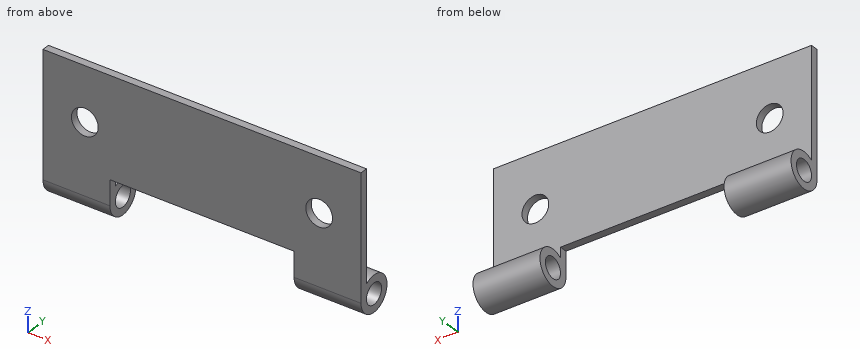
from build123d import *

# Parameters (mm, degrees)
SKETCH_1_R          = 1.25
EXTRUDE_1_DEPTH     = 38
SKETCH_2_R          = 1.6
SKETCH_2_W          = 22
SKETCH_2_H          = 7.890130192
CUT_EXTRUDE_1_DEPTH = 19


with BuildPart() as part:
    # 草图1 → 凸台-拉伸1 (new body)
    with BuildSketch(Plane(origin=(0, 0, 0), x_dir=(0, 0, -1), z_dir=(1, 0, 0))):
        with BuildLine():
            Line((0, -2.15), (-15, -2.15))
            Line((-15, -2.15), (-15, -1.25))
            Line((-15, -1.25), (-1.749285568, -1.25))
            ThreePointArc((-1.749285568, -1.25), (0.983615779, 1.911805429), (0, -2.15))
        make_face()
        Circle(SKETCH_1_R, mode=Mode.SUBTRACT)
    extrude(amount=EXTRUDE_1_DEPTH)

    # 草图2 → 切除-拉伸1 (cut, symmetric)
    with BuildSketch(Plane(origin=(0, 0, 0), x_dir=(1, 0, 0), z_dir=(0, 1, 0))):
        with Locations((33, -8.5)):
            Circle(SKETCH_2_R)
        with Locations((5, -8.5)):
            Circle(SKETCH_2_R)
        with Locations((19, 0.945065096)):
            Rectangle(SKETCH_2_W, SKETCH_2_H)
    extrude(amount=CUT_EXTRUDE_1_DEPTH, both=True, mode=Mode.SUBTRACT)


solid = part.part
Verification items for the finished model (mm, model axes). Give positions to 0.01 mm unless a question says otherwise; leave off trailing zeros. Write each loop counter-clockwise with the first axis right and the second up, starting at its lowest first coordinate (ties: lowest second). Pieces come first, ordered by that corner, then holes. Notation, with made-up numbers: (28.5, 72.25) - (73.5, 72.25) arc R21 ccw to (73.5, 103.25) - close; hole circle Ø8 at (-11.75, 63.5). An arc over 180 degrees is marked (long way). Answer as CSV lines item,"result". Start each with the question number.
1. Sectioned sample at C-C (z = 8.5). Record the boundary of the cut face in (x, y), then the cut area to 3 significant figures.
2. Depth check by flat-ended pin: pin 1 (6 mm diameter, centred on x = 12, z = 6.5, fed in from +Y). Enter the tip coordinate at first touch or a pass-through.
3. Sectioned sample at B-B (y = 0). Record the boundary of the cut face in (x, z).
4. Thickness scan on line 1 (Z direction, x = 36.25, y = 0); line 2 (Z direction, x = 5, y = -1.75); line 3 (Z direction, x = 20, y = -1.6). Record the ranges inside material, lowest first.
5. Sectioned sample at D-D (y = -1.7). Record the boundary of the cut face in (x, z).
6. Sectioned sample at A-A (x = 33). Record the boundary of the cut face in (y, z), then the cut area to 3 significant figures.
Derived:
1,outline,"(0, -2.15) - (3.4, -2.15) - (3.4, -1.25) - (0, -1.25) - close; (6.6, -2.15) - (31.4, -2.15) - (31.4, -1.25) - (6.6, -1.25) - close; (34.6, -2.15) - (38, -2.15) - (38, -1.25) - (34.6, -1.25) - close"
1,area,"28.4 mm²"
2,pin 1,"y = -1.25"
3,outline,"(0, -2.15) - (8, -2.15) - (8, -1.25) - (0, -1.25) - close; (0, 1.25) - (8, 1.25) - (8, 2.15) - (0, 2.15) - close; (30, -2.15) - (38, -2.15) - (38, -1.25) - (30, -1.25) - close; (30, 1.25) - (38, 1.25) - (38, 2.15) - (30, 2.15) - close"
4,line 1,"-2.15 to -1.25, 1.25 to 2.15"
4,line 2,"-1.25 to 6.9, 10.1 to 15"
4,line 3,"3 to 15"
5,outline,"(0, -1.32) - (8, -1.32) - (8, 3) - (30, 3) - (30, -1.32) - (38, -1.32) - (38, 15) - (0, 15) - close; hole circle Ø3.2 at (5, 8.5); hole circle Ø3.2 at (33, 8.5)"
6,outline,"(-2.15, 0) arc R2.15 ccw (long way) to (-1.25, 1.75) - (-1.25, 6.9) - (-2.15, 6.9) - close; (-2.15, 10.1) - (-1.25, 10.1) - (-1.25, 15) - (-2.15, 15) - close; hole circle Ø2.5 at (0, 0)"
6,area,"19.1 mm²"
